```python
from build123d import *

# Parameters (mm, degrees)
SKETCH1_W           = 170
SKETCH1_H           = 220
BOSS_EXTRUDE1_DEPTH = 15
SKETCH2_R           = 2
CUT_EXTRUDE1_DEPTH  = 20
SKETCH3_R           = 3.175
CUT_EXTRUDE2_DEPTH  = 15


with BuildPart() as part:
    # Sketch1 → Boss-Extrude1 (new body)
    with BuildSketch(Plane(origin=(0, 0, 0), x_dir=(1, 0, 0), z_dir=(0, 1, 0))):
        with Locations((85, 110)):
            Rectangle(SKETCH1_W, SKETCH1_H)
    extrude(amount=BOSS_EXTRUDE1_DEPTH)

    # Sketch2 → Cut-Extrude1 (cut)
    with BuildSketch(Plane.ZY):
        with Locations((-10, 7.5)):
            Circle(SKETCH2_R)
        with Locations((-210, 7.5)):
            Circle(SKETCH2_R)
    cut_extrude1 = extrude(amount=-CUT_EXTRUDE1_DEPTH, mode=Mode.SUBTRACT)

    # Sketch3 → Cut-Extrude2 (cut)
    with BuildSketch(Plane(origin=(0, 15, 0), x_dir=(1, 0, 0), z_dir=(0, 1, 0))):
        with Locations((72.5, 15.821244145)):
            Circle(SKETCH3_R)
        with Locations((72.5, 146.891244145)):
            Circle(SKETCH3_R)
    cut_extrude2 = extrude(amount=-CUT_EXTRUDE2_DEPTH, mode=Mode.SUBTRACT)

    # Mirror1: Cut-Extrude1, Cut-Extrude2 across plane
    add(cut_extrude1.mirror(Plane.ZY.offset(-85)), mode=Mode.SUBTRACT)
    add(cut_extrude2.mirror(Plane.ZY.offset(-85)), mode=Mode.SUBTRACT)


solid = part.part
```
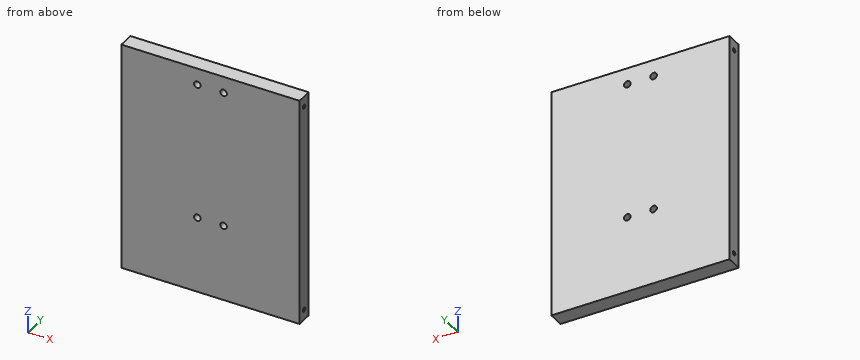
For this review, take the finished solid that the model builds, in its own axes (mm). Round coordinates to 2 decimals unless told otherwise and drop trailing zeros. Write each loop counter-clockwise with the first axis right and the second up, starting at its lowest first coordinate (ties: lowest second). Pieces come first, ordered by that corner, then holes.
1) Take a section at A-A on x = 97.5. Give the boundary of the cut face in (y, z).
Answer below:
outline: (0, -220) - (15, -220) - (15, -150.07) - (0, -150.07) - close; (0, -143.72) - (15, -143.72) - (15, -19) - (0, -19) - close; (0, -12.65) - (15, -12.65) - (15, 0) - (0, 0) - close
2) Insertion check: pin 1 Ø4 at (x, z) = (97.5, -146.89) entering from +Y; pin 2 Ø3 at (y, z) = (7.5, -10) entering from -X; pin 3 Ø1.2 at (y, z) = (8, -11) entering from +X. Each pin has a flat end and moves straight along its axis. Give the tip position at first contact, or say it passes through.
Answer below:
pin 1: passes through
pin 2: stops at x = 20
pin 3: stops at x = 150
3) For line 1 along Z through (x, y) = (97.5, 11); line 2 along Z through (x, y) = (97, 9.5), list the stretches that pass through material, from the lowest coordinate up.
Answer below:
line 1: z = -220 to -150.07, -143.72 to -19, -12.65 to 0
line 2: z = -220 to -150.03, -143.76 to -18.96, -12.69 to 0
